Geometry: final body of the model. Coordinates: model frame, mm. A direction names the side the tool comes from. Coordinates: 2 decimals unless noted, no trailing zeros. Order: outer loops, then holes, each group sorted by start corner. A loop starts at its lowest first (then second) coordinate and runs counter-clockwise, first axis right, second up. Notation, with made-up numbers: (-32.5, 73.5) -> (-28.5, 73.5) arc R22 ccw to (-28.5, 89.5) -> close; hole circle Ø8 at (11, -34). An arc over 180 degrees is marked (long way). Answer in a Markdown table with one row per item. Add a question column.
1) Section query B-B on x = 0. Return the cut outline in (y, z), then the cut area to 3 significant figures.
2) Section query C-C on z = 0.6. Count the separate pieces of the cut face and the enclosed holes in it, then the cut area to 3 significant figures.
3) Section query A-A on y = 22. Return the cut outline in (x, z), then the cut area to 3 significant figures.
4) Set-up query: faces 1 (the face through (14, 4, 1)), 2 (the face through (21, 3.6, 1)), 3 (the face through (11.34, -0.83, 1.01)). Return all of +Z, -Z, +X, -X, +Y, -Y with unobstructed straight access to the full face (end or side cutting, diameter ignored); none if empty.
5) Pull-direction query (X, two-part tool) for faces 4 (the face through (-13.79, 29.32, 0.99)), 5 (the face through (18.7, 26.4, 1)), 6 (the face through (-19.75, 29, 1)), 7 (the face through (-21, 3.6, 1)); classes: +X half, -X half, draft (parallel to the pull), parting line (faces both ways), or undercut.
6) Contact query for flat-ended pins moving along their axis: P1, Ø1, axis at y = -0.5, z = 1.5, coming from the -X side; P2, Ø1, axis at x = -21, z = 1.5, coming from the -Y side; P3, Ø1.6, axis at x = -13.5, y = 28, coming from the +Z side. Output: stop coordinate, or through.
7) Ray query, line 1 (Y direction, x = -13.5, z = 1.6); line 2 (X direction, y = 20, z = 0.9); line 3 (X direction, y = 4.5, z = 0.9). Return the intervals inside material, ascending. Write a range as from..to.
Autodesk Inventor part; units mm, degrees
ref_plane "YZ Plane" through (0, 0, 0) normal (1, 0, 0) x (0, 1, 0)
ref_plane "XZ Plane" through (0, 0, 0) normal (0, 1, 0) x (-1, 0, 0)
ref_plane "XY Plane" through (0, 0, 0) normal (0, 0, 1) x (1, 0, 0)
sketch "スケッチ1" plane through (0, 0, 0) normal (0, 0, 1) x (1, 0, 0)
  circle A0 centre (0, 0) radius 10.5 construction
  line L0 (-13.5, 28) -> (13.5, 28) construction
  line L1 (13.5, 28) -> (13.5, 1) construction
  line L2 (13.5, 1) -> (-13.5, 1) construction
  line L3 (-13.5, 1) -> (-13.5, 28) construction
  line L4 (-13.5, 28) -> (13.5, 1) construction
  line L5 (13.5, 28) -> (-13.5, 1) construction
  line L6 (-13.5, 14.5) -> (13.5, 14.5) construction
  line L7 (0, 28) -> (0, 1) construction
  circle A1 centre (-13.5, 28) radius 1.35
  circle A2 centre (-13.5, 1) radius 2.4 construction
  circle A3 centre (-13.5, 28) radius 2.4 construction
  line L8 (-19.75, 30.4) -> (19.75, 30.4)
  line L9 (-21.75, 25.4) -> (-21.75, 3.6)
  line L10 (-21.75, 25.4) -> (-19.75, 25.4)
  arc A4 (-19.75, 25.4) -> (-19.75, 27.5) centre (-19.75, 26.45) ccw
  line L11 (-19.75, 27.5) -> (-19.75, 30.4)
  line L12 (-21.75, 3.6) -> (-19.75, 3.6)
  arc A5 (-19.75, 1.5) -> (-19.75, 3.6) centre (-19.75, 2.55) ccw
  line L13 (-19.75, 1.5) -> (-19.75, -1.4)
  line L14 (-19.75, -1.4) -> (-10.6584, -1.4)
  line L15 (21.75, 25.4) -> (21.75, 3.6)
  arc A6 (19.75, 27.5) -> (19.75, 25.4) centre (19.75, 26.45) ccw
  line L16 (19.75, 27.5) -> (19.75, 30.4)
  arc A7 (19.75, 3.6) -> (19.75, 1.5) centre (19.75, 2.55) ccw
  line L17 (21.75, 3.6) -> (19.75, 3.6)
  line L18 (19.75, 1.5) -> (19.75, -1.4)
  line L19 (19.75, -1.4) -> (10.6584, -1.4)
  line L20 (21.75, 25.4) -> (19.75, 25.4)
  arc A8 (10.6584, -1.4) -> (-10.6584, -1.4) centre (0, 0) ccw
  circle A9 centre (13.5, 28) radius 1.35
  line L21 (10.5606, 27.4) -> (-10.5606, 27.4)
  arc A10 (-13.5, 25) -> (-10.5606, 27.4) centre (-13.5, 28) ccw
  line L22 (-13.5, 25) -> (-16.75, 25)
  line L23 (-16.75, 25) -> (-16.75, 4)
  arc A11 (12.1063, 4) -> (-12.1063, 4) centre (0, 0) ccw
  line L24 (-16.75, 4) -> (-12.1063, 4)
  arc A12 (10.5606, 27.4) -> (13.5, 25) centre (13.5, 28) ccw
  line L25 (13.5, 25) -> (16.75, 25)
  line L26 (16.75, 25) -> (16.75, 4)
  line L27 (16.75, 4) -> (12.1063, 4)
  line L28 (-13.5, 2.35) -> (-13, 2.35)
  line L29 (-13.5, -0.35) -> (-13, -0.35)
  arc A13 (-13, -0.35) -> (-13, 2.35) centre (-13, 1) ccw
  arc A14 (-13.5, 2.35) -> (-13.5, -0.35) centre (-13.5, 1) ccw
  line L30 (13.5, -0.35) -> (13, -0.35)
  arc A15 (13, 2.35) -> (13, -0.35) centre (13, 1) ccw
  arc A16 (13.5, -0.35) -> (13.5, 2.35) centre (13.5, 1) ccw
  line L31 (13.5, 2.35) -> (13, 2.35)
  point P0 (0, 14.5)
  dimension "d0" = 21
  dimension "d3" = 27
  dimension "d4" = 27
  dimension "d6" = 1
  dimension "d7" = 4.8
  dimension "d8" = 2
  dimension "d9" = 1.05
  dimension "d10" = 39.5
  dimension "d11" = 5
  dimension "d12" = 5
  dimension "d13" = 21.8
  dimension "d14" = 0.25
  dimension "d15" = 3
  dimension "d16" = 3
  dimension "d17" = 3
  dimension "d18" = 2
  dimension "d24" = 2.7
  dimension "d25" = 1.35
  dimension "d26" = 0.5
extrude "押し出し1" add sketch "スケッチ1" along normal blind 2
fillet "フィレット1" radius 2 2 edges at (-10.6584, -1.4, 1) (10.6584, -1.4, 1)
fillet "フィレット2" radius 2 8 edges at (-16.75, 4, 1) (-16.75, 25, 1) (-10.5606, 27.4, 1) (10.5606, 27.4, 1) (16.75, 25, 1) (16.75, 4, 1) (12.1063, 4, 1) (-12.1063, 4, 1)
equation "\"d25\" = 0.5 * d24"
properties part number "Ankle_back_frame" material "アルミニウム 2014-T4"
Result:
| question | item | result |
|---|---|---|
| 1 | outline | (10.75, 0) -> (12.75, 0) -> (12.75, 2) -> (10.75, 2) -> close; (27.4, 0) -> (30.4, 0) -> (30.4, 2) -> (27.4, 2) -> close |
| 1 | area | 10.0 mm2 |
| 2 | separate pieces | 1 |
| 2 | enclosed holes | 5 |
| 2 | area | 499 mm2 |
| 3 | outline | (-21.75, 0) -> (-16.75, 0) -> (-16.75, 2) -> (-21.75, 2) -> close; (16.75, 0) -> (21.75, 0) -> (21.75, 2) -> (16.75, 2) -> close |
| 3 | area | 20.0 mm2 |
| 4 | face 1 | +Z, -Z |
| 4 | face 2 | +Z, -Z, +X, -Y |
| 4 | face 3 | +Z, -Z, -Y |
| 5 | face 4 | undercut |
| 5 | face 5 | +X half |
| 5 | face 6 | -X half |
| 5 | face 7 | draft |
| 6 | P1 | x = -19.75 |
| 6 | P2 | y = 3.6 |
| 6 | P3 | through |
| 7 | line 1 | -1.4..-0.35, 2.35..4, 25..26.65, 29.35..30.4 |
| 7 | line 2 | -21.75..-16.75, 16.75..21.75 |
| 7 | line 3 | -21.75..-16.07, -12.15..-9.76, 9.76..12.15, 16.07..21.75 |
